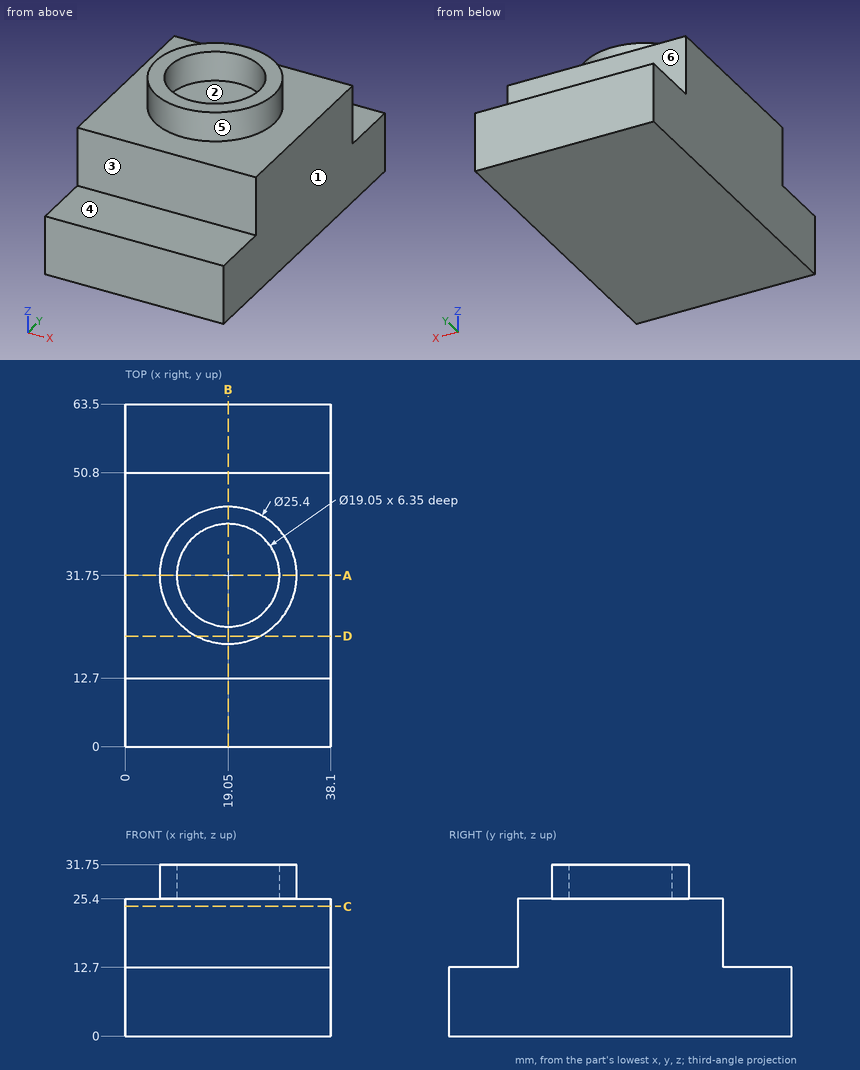
The figure shows three views and two pictorial views of one solid part (mm, origin at its lowest corner). Answer the questions. A direction names the side the tool comes from. Coordinates: 2 decimals unless noted, no trailing zeros. Loops run counter-clockwise (first coordinate to the right, second up) from the corner with the lowest first, then second, coordinate; pieces in that order, holes last. Notation, with made-up numbers: (24.5, 26.5) - (41.5, 26.5) arc R28 ccw to (41.5, 52.5) - close; hole circle Ø11 at (5, 77.25). An arc over 180 degrees is marked (long way). Use a Markdown table: item, result. Add a question column.
1) Given pin 1 (4 mm diameter, centred on x = 13, z = 16, fed in from -Y); pin 2 (8 mm diameter, centred on y = 9, z = 27.5, fed in from -X); pin 3 (5.5 mm diameter, centred on x = 20, y = 32.5, fed in from +Z); pin 4 (6.5 mm diameter, centred on x = 11, y = 57, fed in from +Z), each flat-ended and moving along its own axis, determine where each tip first touches the part or whether it passes through.
2) The part is cut by section A-A, the plane y = 31.75. Give the vertices of the cut face in (x, z) (3 decimals).
3) The part is cut by section D-D, the plane y = 20.5. Give the vertices of the cut face in (x, z), and give its area (3 significant figures).
4) For the marked faces 4, 5 and 6, determine the directions among +Z, -Z, +X, -X, +Y, -Y from which every point of the face is accessible in a straight line to the end or side of a thin tool.
5) The part is cut by section B-B, the plane x = 19.05. Give the vertices of the cut face in (y, z) (3 decimals).
6) Find the intervals of material crossed by line 1 (Y direction, x = 19.05, z = 30.25) (3 decimals); line 2 (Z direction, x = 20, y = 29); line 3 (Y direction, x = 26, z = 15), in increasing order.
7) The mould has two halves that part along X. Classify the marked faces 1, 2 and 3: released by +X, released by -X, zero draft, split by the parting line, or undercut.
8) The part is cut by section C-C, the plane z = 24. Give the vertices of the cut face in (x, y).
Here are the results:
| question | item | result |
|---|---|---|
| 1 | pin 1 | stops at y = 12.7 |
| 1 | pin 2 | passes through |
| 1 | pin 3 | stops at z = 25.4 |
| 1 | pin 4 | stops at z = 12.7 |
| 2 | outline | (0, 0) - (38.1, 0) - (38.1, 25.4) - (31.75, 25.4) - (31.75, 31.75) - (28.575, 31.75) - (28.575, 25.4) - (9.525, 25.4) - (9.525, 31.75) - (6.35, 31.75) - (6.35, 25.4) - (0, 25.4) - close |
| 3 | outline | (0, 0) - (38.1, 0) - (38.1, 25.4) - (24.94, 25.4) - (24.94, 31.75) - (13.16, 31.75) - (13.16, 25.4) - (0, 25.4) - close |
| 3 | area | 1,040 mm^2 |
| 4 | face 4 | +Z, +X, -X, -Y |
| 4 | face 5 | +Z |
| 4 | face 6 | +Z, +X, -X, +Y |
| 5 | outline | (0, 0) - (63.5, 0) - (63.5, 12.7) - (50.8, 12.7) - (50.8, 25.4) - (44.45, 25.4) - (44.45, 31.75) - (41.275, 31.75) - (41.275, 25.4) - (22.225, 25.4) - (22.225, 31.75) - (19.05, 31.75) - (19.05, 25.4) - (12.7, 25.4) - (12.7, 12.7) - (0, 12.7) - close |
| 6 | line 1 | y = 19.05 to 22.225, 41.275 to 44.45 |
| 6 | line 2 | z = 0 to 25.4 |
| 6 | line 3 | y = 12.7 to 50.8 |
| 7 | face 1 | released by +X |
| 7 | face 2 | undercut |
| 7 | face 3 | zero draft |
| 8 | outline | (0, 12.7) - (38.1, 12.7) - (38.1, 50.8) - (0, 50.8) - close |
